```python
from build123d import *

# Parameters (mm, degrees)
SKETCH1_W           = 146.05
SKETCH1_H           = 161.925
BOSS_EXTRUDE1_DEPTH = 3.175
SKETCH2_W           = 19.05
SKETCH2_H           = 3.175
BOSS_EXTRUDE2_DEPTH = 3.175
CUT_EXTRUDE1_DEPTH  = 112.453354172
CUT_EXTRUDE2_REACH  = 113.453
SKETCH4_R           = 1.778


with BuildPart() as part:
    # Sketch1 → Boss-Extrude1 (new body)
    with BuildSketch(Plane(origin=(0, 0, 0), x_dir=(1, 0, 0), z_dir=(0, 1, 0))):
        Rectangle(SKETCH1_W, SKETCH1_H)
    extrude(amount=BOSS_EXTRUDE1_DEPTH)

    # Sketch2 → Boss-Extrude2 (add)
    with BuildSketch(Plane(origin=(0, 3.175, 0), x_dir=(1, 0, 0), z_dir=(0, 1, 0))):
        with Locations((-41.275, 82.55)):
            Rectangle(SKETCH2_W, SKETCH2_H)
        with Locations((41.275, 82.55)):
            Rectangle(SKETCH2_W, SKETCH2_H)
        with Locations((41.275, -82.55)):
            Rectangle(SKETCH2_W, SKETCH2_H)
        with Locations((-41.275, -82.55)):
            Rectangle(SKETCH2_W, SKETCH2_H)
    extrude(amount=-BOSS_EXTRUDE2_DEPTH)

    # Sketch3 → Cut-Extrude1 (cut, through all)
    with BuildSketch(Plane(origin=(0, 3.175, 0), x_dir=(1, 0, 0), z_dir=(0, 1, 0))):
        with BuildLine():
            Line((-57.15, 74.6125), (57.15, 74.6125))
            ThreePointArc((57.15, 74.6125), (63.5, 68.2625), (57.15, 61.9125))
            Line((57.15, 61.9125), (-57.15, 61.9125))
            ThreePointArc((-57.15, 61.9125), (-63.5, 68.2625), (-57.15, 74.6125))
        make_face()
    extrude(amount=-CUT_EXTRUDE1_DEPTH, mode=Mode.SUBTRACT)

    # Sketch4 → Cut-Extrude2 (cut, up to next)
    with BuildSketch(Plane(origin=(0, 3.175, 0), x_dir=(1, 0, 0), z_dir=(0, 1, 0)), mode=Mode.PRIVATE) as cut_extrude2_sk1:
        with Locations(Location((54.229, -55.3085, 0), (0, 0, 270))):
            Circle(SKETCH4_R)
    cut_extrude2_tool1 = extrude(cut_extrude2_sk1.sketch, amount=-CUT_EXTRUDE2_REACH, mode=Mode.PRIVATE) & part.part
    # Sketch4 → Cut-Extrude2 (cut, up to next)
    with BuildSketch(Plane(origin=(0, 3.175, 0), x_dir=(1, 0, 0), z_dir=(0, 1, 0)), mode=Mode.PRIVATE) as cut_extrude2_sk2:
        with Locations(Location((25.273, -55.3085, 0), (0, 0, 270))):
            Circle(SKETCH4_R)
    cut_extrude2_tool2 = extrude(cut_extrude2_sk2.sketch, amount=-CUT_EXTRUDE2_REACH, mode=Mode.PRIVATE) & part.part
    # Sketch4 → Cut-Extrude2 (cut, up to next)
    with BuildSketch(Plane(origin=(0, 3.175, 0), x_dir=(1, 0, 0), z_dir=(0, 1, 0)), mode=Mode.PRIVATE) as cut_extrude2_sk3:
        with Locations(Location((24.4602, -9.2329, 0), (0, 0, 270))):
            Circle(SKETCH4_R)
    cut_extrude2_tool3 = extrude(cut_extrude2_sk3.sketch, amount=-CUT_EXTRUDE2_REACH, mode=Mode.PRIVATE) & part.part
    # Sketch4 → Cut-Extrude2 (cut, up to next)
    with BuildSketch(Plane(origin=(0, 3.175, 0), x_dir=(1, 0, 0), z_dir=(0, 1, 0)), mode=Mode.PRIVATE) as cut_extrude2_sk4:
        with Locations(Location((51.435, -9.2329, 0), (0, 0, 270))):
            Circle(SKETCH4_R)
    cut_extrude2_tool4 = extrude(cut_extrude2_sk4.sketch, amount=-CUT_EXTRUDE2_REACH, mode=Mode.PRIVATE) & part.part
    # Sketch4 → Cut-Extrude2 (cut, up to next)
    with BuildSketch(Plane(origin=(0, 3.175, 0), x_dir=(1, 0, 0), z_dir=(0, 1, 0)), mode=Mode.PRIVATE) as cut_extrude2_sk5:
        with Locations(Location((3.0226, -73.0885, 0), (0, 0, 270))):
            Circle(SKETCH4_R)
    cut_extrude2_tool5 = extrude(cut_extrude2_sk5.sketch, amount=-CUT_EXTRUDE2_REACH, mode=Mode.PRIVATE) & part.part
    # Sketch4 → Cut-Extrude2 (cut, up to next)
    with BuildSketch(Plane(origin=(0, 3.175, 0), x_dir=(1, 0, 0), z_dir=(0, 1, 0)), mode=Mode.PRIVATE) as cut_extrude2_sk6:
        with Locations(Location((-49.911, -73.0885, 0), (0, 0, 270))):
            Circle(SKETCH4_R)
    cut_extrude2_tool6 = extrude(cut_extrude2_sk6.sketch, amount=-CUT_EXTRUDE2_REACH, mode=Mode.PRIVATE) & part.part
    # Sketch4 → Cut-Extrude2 (cut, up to next)
    with BuildSketch(Plane(origin=(0, 3.175, 0), x_dir=(1, 0, 0), z_dir=(0, 1, 0)), mode=Mode.PRIVATE) as cut_extrude2_sk7:
        with Locations(Location((-49.911, -1.2065, 0), (0, 0, 270))):
            Circle(SKETCH4_R)
    cut_extrude2_tool7 = extrude(cut_extrude2_sk7.sketch, amount=-CUT_EXTRUDE2_REACH, mode=Mode.PRIVATE) & part.part
    # Sketch4 → Cut-Extrude2 (cut, up to next)
    with BuildSketch(Plane(origin=(0, 3.175, 0), x_dir=(1, 0, 0), z_dir=(0, 1, 0)), mode=Mode.PRIVATE) as cut_extrude2_sk8:
        with Locations(Location((3.0226, -1.2065, 0), (0, 0, 270))):
            Circle(SKETCH4_R)
    cut_extrude2_tool8 = extrude(cut_extrude2_sk8.sketch, amount=-CUT_EXTRUDE2_REACH, mode=Mode.PRIVATE) & part.part
    # Sketch4 → Cut-Extrude2 (cut, up to next)
    with BuildSketch(Plane(origin=(0, 3.175, 0), x_dir=(1, 0, 0), z_dir=(0, 1, 0)), mode=Mode.PRIVATE) as cut_extrude2_sk9:
        with Locations(Location((-51.689, 10.6807, 0), (0, 0, 270))):
            Circle(SKETCH4_R)
    cut_extrude2_tool9 = extrude(cut_extrude2_sk9.sketch, amount=-CUT_EXTRUDE2_REACH, mode=Mode.PRIVATE) & part.part
    # Sketch4 → Cut-Extrude2 (cut, up to next)
    with BuildSketch(Plane(origin=(0, 3.175, 0), x_dir=(1, 0, 0), z_dir=(0, 1, 0)), mode=Mode.PRIVATE) as cut_extrude2_sk10:
        with Locations(Location((20.2946, 10.6807, 0), (0, 0, 270))):
            Circle(SKETCH4_R)
    cut_extrude2_tool10 = extrude(cut_extrude2_sk10.sketch, amount=-CUT_EXTRUDE2_REACH, mode=Mode.PRIVATE) & part.part
    # Sketch4 → Cut-Extrude2 (cut, up to next)
    with BuildSketch(Plane(origin=(0, 3.175, 0), x_dir=(1, 0, 0), z_dir=(0, 1, 0)), mode=Mode.PRIVATE) as cut_extrude2_sk11:
        with Locations(Location((20.2946, 55.8165, 0), (0, 0, 270))):
            Circle(SKETCH4_R)
    cut_extrude2_tool11 = extrude(cut_extrude2_sk11.sketch, amount=-CUT_EXTRUDE2_REACH, mode=Mode.PRIVATE) & part.part
    add(cut_extrude2_tool1.solids().sort_by_distance((54.229, 3.175, 55.3085))[0], mode=Mode.SUBTRACT)
    add(cut_extrude2_tool2.solids().sort_by_distance((25.273, 3.175, 55.3085))[0], mode=Mode.SUBTRACT)
    add(cut_extrude2_tool3.solids().sort_by_distance((24.4602, 3.175, 9.2329))[0], mode=Mode.SUBTRACT)
    add(cut_extrude2_tool4.solids().sort_by_distance((51.435, 3.175, 9.2329))[0], mode=Mode.SUBTRACT)
    add(cut_extrude2_tool5.solids().sort_by_distance((3.0226, 3.175, 73.0885))[0], mode=Mode.SUBTRACT)
    add(cut_extrude2_tool6.solids().sort_by_distance((-49.911, 3.175, 73.0885))[0], mode=Mode.SUBTRACT)
    add(cut_extrude2_tool7.solids().sort_by_distance((-49.911, 3.175, 1.2065))[0], mode=Mode.SUBTRACT)
    add(cut_extrude2_tool8.solids().sort_by_distance((3.0226, 3.175, 1.2065))[0], mode=Mode.SUBTRACT)
    add(cut_extrude2_tool9.solids().sort_by_distance((-51.689, 3.175, -10.6807))[0], mode=Mode.SUBTRACT)
    add(cut_extrude2_tool10.solids().sort_by_distance((20.2946, 3.175, -10.6807))[0], mode=Mode.SUBTRACT)
    add(cut_extrude2_tool11.solids().sort_by_distance((20.2946, 3.175, -55.8165))[0], mode=Mode.SUBTRACT)


solid = part.part
```
Here's how the part is built. I have some questions about the finished solid (model axes, mm). Give positions to 0.01 mm unless a question says otherwise; leave off trailing zeros. Order: outer loops, then holes, each group sorted by start corner. A loop starts at its lowest first (then second) coordinate and runs counter-clockwise, first axis right, second up. Notation, with made-up numbers: (24.25, -13) - (60.25, -13) arc R25 cw to (60.25, 10) - close; hole circle Ø9 at (81, 21.5). An arc over 180 degrees is marked (long way). Answer as a JSON object with one key per item and string values. Group by question number.
Item 1: For P1, Ø1, axis at y = 1.5, z = 82.5, coming from the +X side; P2, Ø1.6, axis at x = 26.5, y = 1.5, coming from the -Z side; P3, Ø2, axis at x = 54.23, z = 55.31, coming from the +Y side; P4, Ø1, axis at y = 1, z = 83, coming from the -X side, each with a flat end and sliding along its axis, tell me the tip position at first contact or that it passes through.
Item 2: If we section it at B-B on z = -64.5: Please give me the cut outline in (x, y) (3 decimals).
Item 3: If we section it at C-C on y = 1.2: Give the number of separate pieces and of enclosed holes in the cut face, and give its area (3 significant figures).
Item 4: If we section it at A-A on x = -12.5: Please give me the cut outline in (y, z) (1 decimal), and give its area (3 significant figures).
Item 5: If we mould it in two halves opening along Y, with no side actions, what happens to faces 1 (the cylindrical face through (49.858, 1.61, 10.053)), 2 (the flat face through (-1, 0, -1)), 3 (the flat face through (-1, 3.175, -1))? For each: pulls with the +Y half, pulls with the -Y half, needs draft (parallel to the pull), parting line crosses it, or undercut.
Item 6: Please list where these lines run through material, in increasing order: probe 1 along Z at (x, y) = (-55, 2.2); probe 2 along X at (y, z) = (0.4, -56) (3 decimals); probe 3 along Z at (x, y) = (26.5, 2.95).
Result set:
{
 "1": {"P1": "x = 50.8", "P2": "z = -80.96", "P3": "through", "P4": "x = -50.8"},
 "2": {"outline": "(-73.025, 0) - (-62.265, 0) - (-62.265, 3.175) - (-73.025, 3.175) - close; (62.265, 0) - (73.025, 0) - (73.025, 3.175) - (62.265, 3.175) - close"},
 "3": {"separate pieces": "1", "enclosed holes": "12", "area": "22,200 mm²"},
 "4": {"outline": "(0, -81) - (3.2, -81) - (3.2, -74.6) - (0, -74.6) - close; (0, -61.9) - (3.2, -61.9) - (3.2, 81) - (0, 81) - close", "area": "474 mm²"},
 "5": {"face 1": "needs draft", "face 2": "pulls with the -Y half", "face 3": "pulls with the +Y half"},
 "6": {"probe 1": "-80.96 to -74.61, -61.91 to 80.96", "probe 2": "-73.025 to 18.526, 22.063 to 73.025", "probe 3": "-80.96 to -74.61, -61.91 to 54.02, 56.6 to 80.96"}
}
